from build123d import *

# Parameters (mm, degrees)
F1_DEPTH      = 50.8
F3_DEPTH      = 25.4
F3_DEPTH_BACK = 25.4
F4_R          = 3.175
F5_DEPTH      = 1.6129


with BuildPart() as f1:
    # F0 (on Front) → F1 (new body)
    with BuildSketch(Plane.XZ):
        with BuildLine():
            Line((2.2765197791, 8.5634865664), (-9.489294471, 8.5634865664))
            Line((-9.489294471, 8.5634865664), (-9.489294471, 6.9505865664))
            Line((-9.489294471, 6.9505865664), (0, 6.9505865664))
            ThreePointArc((0, 6.9505865664), (0.1429068283, 6.9642762789), (0.2858136566, 6.9505865664))
            ThreePointArc((0.2858136566, 6.9505865664), (0.7644025503, 6.6362301957), (0.8833758177, 6.0761296524))
            Line((0.8833758177, 6.0761296524), (-3.2259208163, -9.4385629753))
            Line((-3.2259208163, -9.4385629753), (-1.6667832808, -9.8515236945))
            Line((-1.6667832808, -9.8515236945), (2.9753029463, 7.6747216416))
            Line((2.9753029463, 7.6747216416), (2.993829025, 7.7446670463))
            ThreePointArc((2.993829025, 7.7446670463), (2.8710717472, 8.2939064661), (2.3770475991, 8.5634865664))
            Line((2.3770475991, 8.5634865664), (2.2765197791, 8.5634865664))
        make_face()
        with BuildLine():
            ThreePointArc((2.3770475991, 8.5634865664), (2.3267836891, 8.5653429014), (2.2765197791, 8.5634865664))
            Line((2.2765197791, 8.5634865664), (2.3770475991, 8.5634865664))
        make_face()
        with BuildLine():
            ThreePointArc((0.2858136566, 6.9505865664), (0.1429068283, 6.9642762789), (0, 6.9505865664))
            Line((0, 6.9505865664), (0.2858136566, 6.9505865664))
        make_face()
        with BuildLine():
            ThreePointArc((2.9753029463, 7.6747216416), (2.9854950368, 7.709448271), (2.993829025, 7.7446670463))
            Line((2.993829025, 7.7446670463), (2.9753029463, 7.6747216416))
        make_face()
    extrude(amount=F1_DEPTH)

    # F2 (on Right) → F3 (cut, two sides)
    with BuildSketch(Plane.YZ) as f3_sk:
        with BuildLine():
            Line((-45.7992069423, -3.3815500792), (-49.0718819201, -9.8507925868))
            Line((-49.0718819201, -9.8507925868), (-37.2894648818, -9.9727063475))
            Line((-37.2894648818, -9.9727063475), (-40.6238138676, -3.3815500792))
            ThreePointArc((-40.6238138676, -3.3815500792), (-43.2115104049, -1.7906479393), (-45.7992069423, -3.3815500792))
        make_face()
        with BuildLine():
            Line((-20.0428648818, -9.9727063475), (-23.3772138676, -3.3815500792))
            ThreePointArc((-23.3772138676, -3.3815500792), (-25.9649104049, -1.7906479393), (-28.5526069423, -3.3815500792))
            Line((-28.5526069423, -3.3815500792), (-31.8252819201, -9.8507925868))
            Line((-31.8252819201, -9.8507925868), (-20.0428648818, -9.9727063475))
        make_face()
        with BuildLine():
            Line((-2.7962648818, -9.9727063475), (-6.1306138676, -3.3815500792))
            ThreePointArc((-6.1306138676, -3.3815500792), (-8.7183104049, -1.7906479393), (-11.3060069423, -3.3815500792))
            Line((-11.3060069423, -3.3815500792), (-14.5786819201, -9.8507925868))
            Line((-14.5786819201, -9.8507925868), (-2.7962648818, -9.9727063475))
        make_face()
    extrude(amount=-F3_DEPTH, mode=Mode.SUBTRACT)
    extrude(f3_sk.sketch, amount=F3_DEPTH_BACK, mode=Mode.SUBTRACT)

    # F4 (on face) → F5 (cut, through all)
    with BuildSketch(Plane.XY.offset(8.5634865664)):
        with Locations((-3.139294471, -7.4458811432)):
            Circle(F4_R)
        with Locations((-3.139294471, -24.7178811432)):
            Circle(F4_R)
        with Locations((-3.139294471, -41.9898811432)):
            Circle(F4_R)
    extrude(amount=-F5_DEPTH, mode=Mode.SUBTRACT)


solid = f1.part
The listing builds one solid part. Answer for the finished solid, in the listing's coordinates (mm). A direction names the side the tool comes from. Coordinates: 2 decimals unless noted, no trailing zeros. Order: outer loops, then holes, each group sorted by start corner. A loop starts at its lowest first (then second) coordinate and runs counter-clockwise, first axis right, second up.
Q1. Which of the six approach directions +Z, -Z, +X, -X, +Y, -Y give full straight-line access (tool end or side, diameter ignored) to faces 4 (the face through (-3.55, -21.57, 7.77)), 5 (the face through (-0.686, -25.044, 0.151)), 6 (the face through (-1.567, -38.964, -6.662))?
Q2. For a pull along Z with two mould halves and no side action, classify faces 1 (the face through (0, -50.8, 1)), 2 (the face through (-0.53, -8.67, -1.79)), 3 (the face through (-7, -25, 6.951)) as pulls with the +Z half, pulls with the -Z half, needs draft (parallel to the pull), parting line crosses it, or undercut.
Q3. A cutting plane is placed at A-A, the plane y = -40. Write down the section's boundary in (x, z), and give its area (3 significant figures).
Q4. A cutting plane is placed at B-B, the plane x = -4.25. Write down the section's boundary in (y, z), and give its area (3 significant figures).
Q5. A cutting plane is placed at C-C, the plane z = -4.75. Write down the section's boundary in (x, y), and give its area (3 significant figures).
Q6. A cutting plane is placed at D-D, the plane y = -19. Write down the section's boundary in (x, z), and give its area (3 significant figures).
Q7. Consider line 1 (Y direction, x = -2, z = -7.25); line 2 (Z direction, x = -4.75, y = -15); line 3 (Y direction, x = -2.5, z = -8.75). Determine where each line is inside the solid, lowest interval first.
Q8. Given P1, Ø4, axis at y = -22, z = -5.5, coming from the +X side; P2, Ø3, axis at x = 0.5, y = -24, coming from the -Z side; P3, Ø6, axis at x = -6.5, y = -9.5, coming from the -Z side, each flat-ended and moving along its own axis, determine where each tip first touches the part or whether it passes through.
Answers follow:
1. face 4: +Z
1. face 5: -X, +Y, -Y
1. face 6: -Z, +X, -X
2. face 1: needs draft
2. face 2: pulls with the -Z half
2. face 3: undercut
3. outline: (-9.49, 6.95) - (-5.61, 6.95) - (-5.61, 8.56) - (-9.49, 8.56) - close; (-1.95, -4.61) - (-0.28, -4.61) - (2.98, 7.67) arc R0.68 ccw to (2.28, 8.56) - (-0.67, 8.56) - (-0.67, 6.95) - (0.29, 6.95) arc R0.75 cw to (0.88, 6.08) - close
3. area: 31.5 mm2
4. outline: (-50.8, 6.95) - (-44.96, 6.95) - (-44.96, 8.56) - (-50.8, 8.56) - close; (-39.02, 6.95) - (-27.69, 6.95) - (-27.69, 8.56) - (-39.02, 8.56) - close; (-21.74, 6.95) - (-10.42, 6.95) - (-10.42, 8.56) - (-21.74, 8.56) - close; (-4.47, 6.95) - (0, 6.95) - (0, 8.56) - (-4.47, 8.56) - close
4. area: 53.2 mm2
5. outline: (-1.98, -50.8) - (-0.32, -50.8) - (-0.32, -46.49) - (-1.98, -46.49) - close; (-1.98, -39.93) - (-0.32, -39.93) - (-0.32, -29.24) - (-1.98, -29.24) - close; (-1.98, -22.68) - (-0.32, -22.68) - (-0.32, -12) - (-1.98, -12) - close; (-1.98, -5.44) - (-0.32, -5.44) - (-0.32, 0) - (-1.98, 0) - close
5. area: 51.9 mm2
6. outline: (-9.49, 6.95) - (0.29, 6.95) arc R0.75 cw to (0.88, 6.08) - (-3.23, -9.44) - (-1.67, -9.85) - (2.98, 7.67) arc R0.68 ccw to (2.28, 8.56) - (-9.49, 8.56) - close
6. area: 47.9 mm2
7. line 1: y = -50.8 to -47.76, -38.67 to -30.51, -21.42 to -13.26, -4.17 to 0
7. line 2: z = 6.95 to 8.56
7. line 3: y = -50.8 to -48.52, -37.91 to -31.27, -20.66 to -14.02, -3.41 to 0
8. P1: stops at x = 0.02
8. P2: stops at z = -4.67
8. P3: stops at z = 6.95
